Can you work these out from the model? Positions are in its coordinate system, mm. Round coordinates to 2 decimals unless told otherwise and drop trailing zeros. Write each loop counter-clockwise with the first axis right and the second up, starting at its lowest first coordinate (ties: lowest second). Pieces come first, ordered by that corner, then holes. Notation, with made-up numbers: (53, -2.75) -> (97, -2.75) arc R19 cw to (97, 30.25) -> close; hole circle Ø4 at (86.5, 71). An arc over 180 degrees is marked (long way). Write item = value, one per line. Start each with the question number.
1) Thinking about a two-plate mould opening in X: for faces 1 (the face through (221, 217, 0)), 2 (the face through (455.132, 508.444, 0.74)), 3 (the face through (298.409, -117.567, 0.74)), 4 (the face through (-62.562, 200.213, 0.74)), which applies, +X half, -X half, draft (parallel to the pull), parting line (faces both ways), or undercut?
2) If I drill on line 1 (Y direction, x = 120.5, z = 0.3); line 2 (Y direction, x = 206.5, z = 1.4); line 3 (X direction, y = 452, z = 0.1), over which ranges is the centre line in solid material (lowest first)?
3) Imagine slicing it at A-A, the plane z = 0.75. Please give me the cut outline in (x, y) (3 decimals).
4) Imagine slicing it at B-B, the plane y = -24. Please give me the cut outline in (x, z).
5) Imagine slicing it at C-C, the plane x = 122. Please give me the cut outline in (y, z), then the cut area to 3 significant figures.
from build123d import *

# Parameters (mm, degrees)
BOSS_EXTRUDE1_DEPTH = 1.5


with BuildPart() as part:
    # Sketch1 → Boss-Extrude1 (new body)
    with BuildSketch(Plane.XY):
        with BuildLine():
            Line((100.41499283, 808.450676409), (265.41499283, 808.450676409))
            Line((265.41499283, 808.450676409), (650.236066342, 199.917405846))
            Line((650.236066342, 199.917405846), (650.236066342, -391.229199842))
            Line((650.236066342, -391.229199842), (600.236066342, -391.229199842))
            ThreePointArc((600.236066342, -391.229199842), (292.098902578, -117.502355805), (-16.038261187, -391.229199842))
            Line((-16.038261187, -391.229199842), (-221.038261187, -391.229199842))
            Line((-221.038261187, -391.229199842), (100.41499283, 808.450676409))
        make_face()
    extrude(amount=BOSS_EXTRUDE1_DEPTH)


solid = part.part
Reported:
q1.face_1 = draft
q1.face_2 = +X half
q1.face_3 = undercut
q1.face_4 = -X half
q2.line_1 = -169.27 to 808.45
q2.line_2 = -129.54 to 808.45
q2.line_3 = 4.9 to 490.83
q3.outline = (-221.038, -391.229) -> (-16.038, -391.229) arc R310.3 cw to (600.236, -391.229) -> (650.236, -391.229) -> (650.236, 199.917) -> (265.415, 808.451) -> (100.415, 808.451) -> close
q4.outline = (-122.64, 0) -> (650.24, 0) -> (650.24, 1.5) -> (-122.64, 1.5) -> close
q5.outline = (-168.28, 0) -> (808.45, 0) -> (808.45, 1.5) -> (-168.28, 1.5) -> close
q5.area = 1,470 mm²
